```python
from build123d import *

# Parameters (mm, degrees)
MAINBLOCK_DEPTH     = 3.81
BOSS_EXTRUDE1_DEPTH = 19.05
SKETCH3_R           = 1.0795
CUT_EXTRUDE1_DEPTH  = 125.757705173


with BuildPart() as part:
    # Sketch1 → MainBlock (new body)
    with BuildSketch(Plane(origin=(0, 0, 0), x_dir=(1, 0, 0), z_dir=(0, 1, 0))):
        with BuildLine():
            Line((-95.25, 22.479), (95.25, 22.479))
            ThreePointArc((95.25, 22.479), (117.729, 0), (95.25, -22.479))
            Line((95.25, -22.479), (-95.25, -22.479))
            ThreePointArc((-95.25, -22.479), (-117.729, 0), (-95.25, 22.479))
        make_face()
    extrude(amount=MAINBLOCK_DEPTH)

    # Sketch2 → Boss-Extrude1 (add)
    with BuildSketch(Plane.XZ):
        with BuildLine():
            Line((-95.25, 25.4), (95.25, 25.4))
            ThreePointArc((95.25, 25.4), (120.65, 0), (95.25, -25.4))
            Line((95.25, -25.4), (-95.25, -25.4))
            ThreePointArc((-95.25, -25.4), (-120.65, 0), (-95.25, 25.4))
        make_face()
        with BuildLine():
            Line((95.25, 22.479), (-95.25, 22.479))
            ThreePointArc((-95.25, 22.479), (-117.729, 0), (-95.25, -22.479))
            Line((-95.25, -22.479), (95.25, -22.479))
            ThreePointArc((95.25, -22.479), (117.729, 0), (95.25, 22.479))
        make_face(mode=Mode.SUBTRACT)
    extrude(amount=-BOSS_EXTRUDE1_DEPTH)

    # Sketch3 → Cut-Extrude1 (cut, through all)
    with BuildSketch(Plane.XZ):
        with Locations(Location((0, 0, 0), (0, 0, 270))):
            Circle(SKETCH3_R)
        with Locations(Location((-64.77, 0, 0), (0, 0, 270))):
            Circle(SKETCH3_R)
        with Locations(Location((64.77, 0, 0), (0, 0, 270))):
            Circle(SKETCH3_R)
    extrude(amount=-CUT_EXTRUDE1_DEPTH, mode=Mode.SUBTRACT)


solid = part.part
```
CAD build for the part. Positions are in the model's coordinates, mm. A direction names the side the tool comes from. Give positions to 0.01 mm unless a question says otherwise; leave off trailing zeros. Write each loop counter-clockwise with the first axis right and the second up, starting at its lowest first coordinate (ties: lowest second). Pieces come first, ordered by that corner, then holes. Notation, with made-up numbers: M 16.25,31 L 54.25,31 A18 ccw 54.25,46 Z; hole C 20,55 d7. An arc over 180 degrees is marked long. Return JSON: item names as keys, results as strings. Group by question number.
(1) 3-axis set-ups, long thin cutter, end or side, ignore diameter. For faces 5 (the face through (-117.724, 11.323, 0.494)), 6 (the face through (-1, 9, 25.4)): which of +Z, -Z, +X, -X, +Y, -Y reach the whole face in a straight line?
(2) Mould opens along X. For faces 1 (the face through (1, 19.05, 23)), 2 (the face through (120.644, 9.392, 0.559)), 3 (the face through (1, 11, 22.479)), 4 (the face through (-120.644, 9.392, -0.559)) say: pulls with the +X half, pulls with the -X half, needs draft (parallel to the pull), parting line crosses it, or undercut.
(3) Band-saw the part on C-C (z = -19). Give the cut face in (x, y), and give its area (3 significant figures).
(4) Drill centre lines: L1, parallel to X at y = 1.15, z = 0; L2, parallel to Z at x = 64.77, y = 2.6; L3, parallel to Z at x = 63, y = 12.5. Where is each one in solid material? Low to high. Write a range as [from, to].
(5) Band-saw the part on B-B (x = -59.5). Give the cut face in (y, z), and give its area (3 significant figures).
(6) Band-saw the part on A-A (y = 16). Give the cut face in (x, z).
(7) Flat gauge pins, fed straight in: pin 1 Ø3 at (x, z) = (0, 0) entering from +Y; pin 2 Ø2 at (y, z) = (17, 6) entering from +X; pin 3 Ø8 at (y, z) = (17, 9.5) entering from +X. Where does each tip first touch, or does it go through?
Entries:
{
 "1": {"face 5": "+Y", "face 6": "+Z, +X, -X, +Y, -Y"},
 "2": {"face 1": "needs draft", "face 2": "pulls with the +X half", "face 3": "undercut", "face 4": "pulls with the -X half"},
 "3": {"outline": "M -112.11,0 L 112.11,0 L 112.11,19.05 L 107.26,19.05 L 107.26,3.81 L -107.26,3.81 L -107.26,19.05 L -112.11,19.05 Z", "area": "1,000 mm^2"},
 "4": {"L1": "x = [-120.65, -65.85], [-63.69, -1.08], [1.08, 63.69], [65.85, 120.65]", "L2": "z = [-25.4, -1.08], [1.08, 25.4]", "L3": "z = [-25.4, -22.48], [22.48, 25.4]"},
 "5": {"outline": "M 0,-25.4 L 19.05,-25.4 L 19.05,-22.48 L 3.81,-22.48 L 3.81,22.48 L 19.05,22.48 L 19.05,25.4 L 0,25.4 Z", "area": "283 mm^2"},
 "6": {"outline": "M -95.25,-25.4 L 95.25,-25.4 A25.4 ccw 95.25,25.4 L -95.25,25.4 A25.4 ccw Z; hole M -95.25,-22.48 L 95.25,-22.48 A22.48 ccw 95.25,22.48 L -95.25,22.48 A22.48 ccw Z"},
 "7": {"pin 1": "stops at y = 3.81", "pin 2": "stops at x = 120.15", "pin 3": "stops at x = 120.05"}
}
